CAD build for the part. Positions are in the model's coordinates, mm. A direction names the side the tool comes from. Round coordinates to 2 decimals unless told otherwise and drop trailing zeros. Loops run counter-clockwise (first coordinate to the right, second up) from the corner with the lowest first, then second, coordinate; pieces in that order, holes last. Notation, with made-up numbers: (-34.5, 82) -> (-10.5, 82) arc R25 cw to (-10.5, 106) -> close; hole circle Ø4 at (-17, 77.5). An arc over 180 degrees is marked (long way). Answer as CSV lines item,"result".
```python
from build123d import *

# Parameters (mm, degrees)
SKETCH_R   = 16
SKETCH_R_2 = 6.25
PAD_DEPTH  = 8


with BuildPart() as part:
    # Sketch → Pad (new body)
    with BuildSketch(Plane.XY):
        with BuildLine():
            ThreePointArc((-32, 0), (-22.627417, -22.627417), (0, -32))
            Line((0, -32), (210, -32))
            ThreePointArc((210, -32), (242, 0), (210, 32))
            Line((45, 32), (210, 32))
            ThreePointArc((15, 62), (23.786797, 40.786797), (45, 32))
            Line((15, 100), (15, 62))
            ThreePointArc((15, 100), (10.606602, 110.606602), (0, 115))
            Line((0, 115), (-0.1, 115))
            ThreePointArc((-0.1, 115), (-9.335368, 111.819813), (-14.65471, 103.62773))
            Line((-14.65471, 103.62773), (-31.55471, 35.82373))
            ThreePointArc((-31.55471, 35.82373), (-31.888261, 34.023479), (-32, 32.196))
            Line((-32, 32.196), (-32, 0))
        make_face()
        Circle(SKETCH_R, mode=Mode.SUBTRACT)
        with Locations((70, 0)):
            Circle(SKETCH_R_2, mode=Mode.SUBTRACT)
        with Locations((140, 0)):
            Circle(SKETCH_R_2, mode=Mode.SUBTRACT)
        with Locations((210, 0)):
            Circle(SKETCH_R_2, mode=Mode.SUBTRACT)
        with BuildLine():
            ThreePointArc((-1.447096, 105.046624), (-5.046624, 98.552904), (1.447096, 94.953376))
            ThreePointArc((1.447096, 94.953376), (5.046624, 101.447096), (-1.447096, 105.046624))
        make_face(mode=Mode.SUBTRACT)
    extrude(amount=PAD_DEPTH)


solid = part.part
```
Q1. Slice it at B-B, the plane z = 4.5. Give the cut face in (x, y), and give its area (3 significant figures).
Results:
outline,"(-32, 0) arc R32 ccw to (0, -32) -> (210, -32) arc R32 ccw to (210, 32) -> (45, 32) arc R30 cw to (15, 62) -> (15, 100) arc R15 ccw to (0, 115) -> (-0.1, 115) arc R15 ccw to (-14.65, 103.63) -> (-31.55, 35.82) arc R15 ccw to (-32, 32.2) -> close; hole circle Ø32 at (0, 0); hole circle Ø10.5 at (0, 100); hole circle Ø12.5 at (70, 0); hole circle Ø12.5 at (140, 0); hole circle Ø12.5 at (210, 0)"
area,"18,800 mm2"
Q2. Tool access for faces 4 (the cylindrical face through (-3.47, -15.62, 3.94)), 5 (the flat face through (126, 32, 4)): list every direction of +Z, -Z, +X, -X, +Y, -Y with a clear straight run to the whole face (end or side of a thin tool).
Results:
face 4,"+Z, -Z"
face 5,"+Z, -Z, +X, +Y"
Q3. Slice it at A-A, the plane x = 70. Give the cut face in (y, z), and give its area (3 significant figures).
Results:
outline,"(-32, 0) -> (-6.25, 0) -> (-6.25, 8) -> (-32, 8) -> close; (6.25, 0) -> (32, 0) -> (32, 8) -> (6.25, 8) -> close"
area,"412 mm2"
Q4. Slice it at C-C, the plane x = 163. Give the cut face in (y, z).
Results:
outline,"(-32, 0) -> (32, 0) -> (32, 8) -> (-32, 8) -> close"
Q5. Slice it at D-D, the plane y = 21. Give the cut face in (x, z), and give its area (3 significant figures).
Results:
outline,"(-32, 0) -> (234.15, 0) -> (234.15, 8) -> (-32, 8) -> close"
area,"2,130 mm2"
Q6. Probe L1, parallel to X at y = 1, z = 6.5; L2, parallel to Y at x = 210, z = 5.5; L3, parallel to X at y = 2.5, z = 3.5. List the from-to ranges inside material, lowest first. Write a range as [from, to].
Results:
L1,"[-32, -15.97], [15.97, 63.83], [76.17, 133.83], [146.17, 203.83], [216.17, 241.98]"
L2,"[-32, -6.25], [6.25, 32]"
L3,"[-32, -15.8], [15.8, 64.27], [75.73, 134.27], [145.73, 204.27], [215.73, 241.9]"
Q7. Two-plate mould, pull along X, no slides. Class faces 1 (the flat face through (-22.986, 70.2, 3.944)), 2 (the cylindrical face through (75.96, 1.88, 3.94)), 3 (the flat face through (15, 81, 4)): pulls with the +X half, pulls with the -X half, needs draft (parallel to the pull), parting line crosses it, or undercut.
Results:
face 1,"pulls with the -X half"
face 2,"undercut"
face 3,"pulls with the +X half"
Q8. Drop flat-ended pins along their axis: pin 1 Ø1 at (y, z) = (66, 1.5) entering from -X; pin 2 Ø3 at (x, z) = (121.5, 2.5) entering from +Y; pin 3 Ø4 at (x, z) = (5, 3) entering from +Y. Give the stop position or say it passes through.
Results:
pin 1,"x = -24.16"
pin 2,"y = 32"
pin 3,"y = 114.7"
